Here's how the part is built. I have some questions about the finished solid (model axes, mm). Round coordinates to 2 decimals unless told otherwise and drop trailing zeros. Order: outer loops, then holes, each group sorted by start corner. A loop starts at its lowest first (then second) coordinate and runs counter-clockwise, first axis right, second up.
```python
from build123d import *

# Parameters (mm, degrees)
SKETCH1_W                 = 60
SKETCH1_H                 = 45
BOSS_EXTRUDE1_DEPTH       = 2
F_3_0MM_DOWEL_HOLE1_D     = 3
F_3_0MM_DOWEL_HOLE1_DEPTH = 20
F_3_0MM_DOWEL_HOLE1_TIP   = 0.901290929
FILLET2_R                 = 1
FILLET1_R                 = 1
SKETCH4_R                 = 1.75
SKETCH4_W                 = 4.3
SKETCH4_H                 = 10.5
CUT_EXTRUDE1_DEPTH        = 3


with BuildPart() as part:
    # Sketch1 → Boss-Extrude1 (new body)
    with BuildSketch(Plane(origin=(0, 0, 0), x_dir=(0, 0, -1), z_dir=(1, 0, 0))):
        Rectangle(SKETCH1_W, SKETCH1_H)
    extrude(amount=BOSS_EXTRUDE1_DEPTH)

    # Ø3.0mm Dowel Hole1
    with Locations(Plane(origin=(2, 0, 0), x_dir=(0, 0, -1), z_dir=(1, 0, 0))):
        with Locations((-27.5, 20), (27.5, 20), (27.5, -20), (-27.5, -20)):
            Hole(F_3_0MM_DOWEL_HOLE1_D / 2, depth=F_3_0MM_DOWEL_HOLE1_DEPTH)
            with Locations((0, 0, -(F_3_0MM_DOWEL_HOLE1_DEPTH + F_3_0MM_DOWEL_HOLE1_TIP / 2))):  # 118° drill point
                Cone(0, F_3_0MM_DOWEL_HOLE1_D / 2, F_3_0MM_DOWEL_HOLE1_TIP, mode=Mode.SUBTRACT)

    # Fillet2
    fillet2_edges = [part.edges().sort_by_distance(p)[0] for p in [
        (1, -22.5, -30),
        (1, -22.5, 30),
        (1, 22.5, 30),
        (1, 22.5, -30),
    ]]
    fillet(fillet2_edges, radius=FILLET2_R)

    # Fillet1
    fillet1_edges = [part.edges().sort_by_distance(p)[0] for p in [
        (2, 0, -30),
        (2, -22.5, 0),
        (2, 22.5, 0),
        (2, 0, 30),
        (2, 22.207106781, 29.707106781),
        (2, 22.207106781, -29.707106781),
        (2, -22.207106781, 29.707106781),
        (2, -22.207106781, -29.707106781),
    ]]
    fillet(fillet1_edges, radius=FILLET1_R - 0.0001)  # a hair under: the kernel refuses the full size

    # Sketch4 → Cut-Extrude1 (cut)
    with BuildSketch(Plane(origin=(2, 0, 0), x_dir=(0, 0, -1), z_dir=(1, 0, 0))):
        with Locations((-19, 10.75)):
            Circle(SKETCH4_R)
        with Locations((-19, -4.5)):
            Rectangle(SKETCH4_W, SKETCH4_H)
    extrude(amount=-CUT_EXTRUDE1_DEPTH, mode=Mode.SUBTRACT)


solid = part.part
```
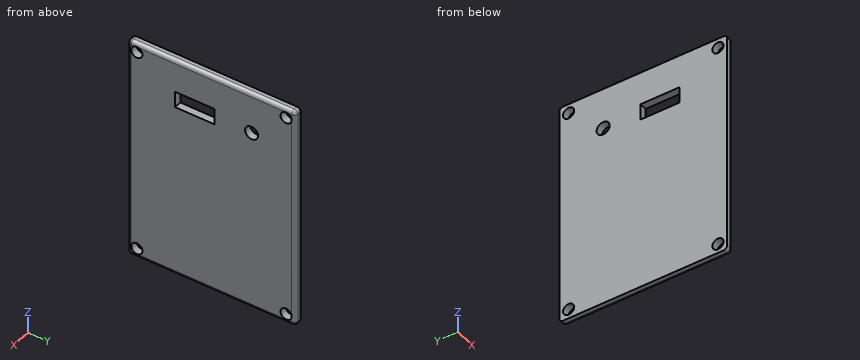
1) I'm going to push flat-ended pins straight in: pin 1 (5 mm diameter, centred on y = 1.5, z = 4.5, fed in from -X); pin 2 (2.5 mm diameter, centred on y = -20, z = 27.5, fed in from +X). Where does each tip first touch, or does it pass through?
2) If we section it at C-C (y = -4.5): Write out the boundary of the cut face in (x, z), plus the area to 3 significant figures.
3) If we section it at D-D (x = 0.6): Write out the boundary of the cut face in (y, z).
4) If we section it at A-A (y = 20): Give the number of separate pieces and of enclosed holes in the cut face, plus the area to 3 significant figures.
5) I need wall thicknesses on line 1 (Y direction, x = 0.75, z = 19); line 2 (Y direction, x = 0.75, z = 27.5); line 3 (Z direction, x = 0.8, y = 0). Which ranges of each line are inside material? Lowest first, please.
Solutions:
1. pin 1: stops at x = 0
1. pin 2: passes through
2. outline: (0, -30) - (1, -30) arc R1 ccw to (2, -29) - (2, 16.85) - (0, 16.85) - close; (0, 21.15) - (2, 21.15) - (2, 29) arc R1 ccw to (1, 30) - (0, 30) - close
2. area: 111 mm2
3. outline: (-22.5, -29) arc R1 ccw to (-21.5, -30) - (21.5, -30) arc R1 ccw to (22.5, -29) - (22.5, 29) arc R1 ccw to (21.5, 30) - (-21.5, 30) arc R1 ccw to (-22.5, 29) - close; hole circle Ø3 at (-20, -27.5); hole circle Ø3 at (-20, 27.5); hole (-9.75, 16.85) - (0.75, 16.85) - (0.75, 21.15) - (-9.75, 21.15) - close; hole circle Ø3.5 at (10.75, 19); hole circle Ø3 at (20, -27.5); hole circle Ø3 at (20, 27.5)
4. separate pieces: 3
4. enclosed holes: 0
4. area: 108 mm2
5. line 1: y = -22.5 to -9.75, 0.75 to 9, 12.5 to 22.5
5. line 2: y = -22.5 to -21.5, -18.5 to 18.5, 21.5 to 22.5
5. line 3: z = -30 to 16.85, 21.15 to 30
